Model file for the job. Use its own axes, mm. Coordinates: 2 decimals unless noted, no trailing zeros. Write each loop counter-clockwise with the first axis right and the second up, starting at its lowest first coordinate (ties: lowest second). Pieces come first, ordered by that corner, then holes.
Q1. Band-saw the part on C-C, the plane z = 25. Write the cut outline in (x, y).
Q2. Drill centre lines: probe 1 along X at (y, z) = (-2.75, 25); probe 2 along X at (y, z) = (-4, 1). Where is each one in solid material? Low to high.
Q3. Pull direction Z, two halves, no side cores. Call faces 1 (the cylindrical face through (-87.59, -3.22, 25.57)), 2 (the cylindrical face through (-94, -3, -33)), 3 (the flat face through (-1, 0, 7)): released by +Z, released by -Z, zero draft, split by the parting line, or undercut.
Q4. Band-saw the part on D-D, the plane x = 60. Write the cut outline in (y, z), plus the area to 3 significant figures.
Q5. Band-saw the part on A-A, the plane x = 85. Write the cut outline in (y, z), plus the area to 3 significant figures.
Q6. Band-saw the part on B-B, the plane z = 0. Write the cut outline in (x, y), plus the area to 3 significant figures.
from build123d import *

# Parameters (mm, degrees)
SKETCH1_W            = 190
SKETCH1_H            = 70
BOSS_EXTRUDE1_DEPTH  = 6.35
M5_CLEARANCE_HOLE1_D = 5.3
FILLET1_R            = 5


with BuildPart() as part:
    # Sketch1 → Boss-Extrude1 (new body)
    with BuildSketch(Plane(origin=(0, 0, 0), x_dir=(1, 0, 0), z_dir=(0, 1, 0))):
        Rectangle(SKETCH1_W, SKETCH1_H)
    extrude(amount=-BOSS_EXTRUDE1_DEPTH)

    # M5 Clearance Hole1 (through all)
    with Locations(Plane(origin=(-85, 0, -25), x_dir=(0, 0, 1), z_dir=(0, 1, 0))):
        with Locations((0, 0), (50, 0), (25, 145), (0, 170), (25, 85), (25, 25), (50, 170)):
            Hole(M5_CLEARANCE_HOLE1_D / 2)

    # Fillet1
    fillet1_edges = [part.edges().sort_by_distance(p)[0] for p in [
        (-95, -3.175, -35),
        (95, -3.175, -35),
        (95, -3.175, 35),
        (-95, -3.175, 35),
    ]]
    fillet(fillet1_edges, radius=FILLET1_R)


solid = part.part
Answer sheet:
1. outline: (-95, -6.35) - (-87.65, -6.35) - (-87.65, 0) - (-95, 0) - close; (-82.35, -6.35) - (82.35, -6.35) - (82.35, 0) - (-82.35, 0) - close; (87.65, -6.35) - (95, -6.35) - (95, 0) - (87.65, 0) - close
2. probe 1: x = -95 to -87.65, -82.35 to 82.35, 87.65 to 95
2. probe 2: x = -95 to -62.45, -57.55 to -2.45, 2.45 to 57.55, 62.45 to 95
3. face 1: undercut
3. face 2: released by -Z
3. face 3: zero draft
4. outline: (-6.35, -35) - (0, -35) - (0, -2.65) - (-6.35, -2.65) - close; (-6.35, 2.65) - (0, 2.65) - (0, 35) - (-6.35, 35) - close
4. area: 411 mm2
5. outline: (-6.35, -35) - (0, -35) - (0, -27.65) - (-6.35, -27.65) - close; (-6.35, -22.35) - (0, -22.35) - (0, 22.35) - (-6.35, 22.35) - close; (-6.35, 27.65) - (0, 27.65) - (0, 35) - (-6.35, 35) - close
5. area: 377 mm2
6. outline: (-95, -6.35) - (-62.65, -6.35) - (-62.65, 0) - (-95, 0) - close; (-57.35, -6.35) - (-2.65, -6.35) - (-2.65, 0) - (-57.35, 0) - close; (2.65, -6.35) - (57.35, -6.35) - (57.35, 0) - (2.65, 0) - close; (62.65, -6.35) - (95, -6.35) - (95, 0) - (62.65, 0) - close
6. area: 1,110 mm2
